Autodesk Inventor part; units mm, degrees
ref_plane "Work Plane3" through (-28.9586, -30.6315, -38.1) normal (-0.9063, 0.4226, 0) x (0, 0, 1)
ref_plane "Work Plane4" through (30.6491, -34.2567, 0.3) normal (0.9063, 0.4226, 0) x (0, 0, -1)
ref_plane "YZ Plane" through (0, 0, 0) normal (1, 0, 0) x (0, 1, 0)
sketch "Sketch19" plane through (0, 0, 0) normal (0, 0, 1) x (1, 0, 0)
  line L0 (47.55, -58) -> (-47.55, -58)
  line L1 (-100, -14) -> (156, -14) construction
  arc A0 (47.55, -58) -> (73.6817, -14) centre (0, 0) ccw
  arc A1 (-73.6817, -14) -> (-47.55, -58) centre (0, 0) ccw
  arc A2 (-64.7514, -20.7668) -> (-73.3933, -15.4412) centre (-66.5432, -14) ccw
  arc A3 (73.3933, -15.4412) -> (64.7514, -20.7668) centre (66.5432, -14) ccw
  arc A4 (-67.6299, -7.0849) -> (-64.8992, -20.3) centre (0, 0) ccw construction
  arc A5 (-64.7514, -20.7668) -> (-46.0869, -50) centre (0, 0) ccw
  arc A6 (46.0869, -50) -> (64.7514, -20.7668) centre (0, 0) ccw
  arc A7 (64.8058, -20.5962) -> (67.6299, -7.0849) centre (0, 0) ccw construction
  line L2 (0, 0) -> (-33.9351, 15.8242) construction
  line L3 (0, 0) -> (37.291, 17.3891) construction
  line L4 (0, 0) -> (0, -41) construction
  line L5 (0, 0) -> (-21.2237, -45.5143) construction
  line L6 (0, 0) -> (17.7082, -37.9755) construction
  line L7 (-12, -38.5394) -> (-12, -50)
  line L8 (12, -38.5394) -> (12, -50)
  line L9 (-26, -32.0111) -> (-26, -50)
  line L10 (26, -32.0111) -> (26, -50)
  line L11 (-18.4455, -35.5339) -> (-20.1359, -39.1591)
  line L12 (-20.1359, -39.1591) -> (-17.0545, -40.596)
  line L13 (-17.0545, -40.596) -> (-15.364, -36.9708)
  line L14 (15.364, -36.9708) -> (17.0545, -40.596)
  line L15 (17.0545, -40.596) -> (20.1359, -39.1591)
  line L16 (20.1359, -39.1591) -> (18.4455, -35.5339)
  line L17 (-12, -38.5394) -> (-15.364, -36.9708)
  line L18 (-18.4455, -35.5339) -> (-26, -32.0111)
  line L19 (12, -38.5394) -> (15.364, -36.9708)
  line L20 (18.4455, -35.5339) -> (26, -32.0111)
  line L21 (-46.0869, -50) -> (-26, -50)
  line L22 (-12, -50) -> (12, -50)
  line L23 (26, -50) -> (46.0869, -50)
  dimension "d378" = 58
  dimension "d379" = 14
  dimension "d381" = 75
  dimension "d383" = 75
  dimension "d384" = 14
  dimension "d385" = 14
  dimension "d389" = 25
  dimension "d390" = 25
  dimension "d391" = 90
  dimension "d392" = 90
  dimension "d393" = 24
  dimension "d394" = 12
  dimension "d395" = 14
  dimension "d396" = 14
  dimension "d399" = 3.4
  dimension "d400" = 4
  dimension "d401" = 1.7
  dimension "d402" = 3.4
  dimension "d403" = 1.7
  dimension "d404" = 4
extrude "Extrusion17" add sketch "Sketch19" along normal blind 140
sketch "Sketch20" plane through (0, 0, 0) normal (0, 0, -1) x (-1, 0, 0)
  line L0 (74, -50) -> (74, -58)
  line L1 (74, -58) -> (-74, -58)
  line L2 (-74, -58) -> (-74, -50)
  line L3 (47.55, -58) -> (-47.55, -58)
  line L4 (26, -50) -> (46.0869, -50)
  line L5 (-46.0869, -50) -> (-26, -50)
  line L6 (-26, -50) -> (-26, -32.0111)
  line L7 (-26, -32.0111) -> (-18.4455, -35.5339)
  line L8 (-18.4455, -35.5339) -> (-20.1359, -39.1591)
  line L9 (-20.1359, -39.1591) -> (-17.0545, -40.596)
  line L10 (-17.0545, -40.596) -> (-15.364, -36.9708)
  line L11 (-15.364, -36.9708) -> (-12, -38.5394)
  line L12 (-12, -38.5394) -> (-12, -50)
  line L13 (-12, -50) -> (12, -50)
  line L14 (12, -50) -> (12, -38.5394)
  line L15 (12, -38.5394) -> (15.364, -36.9708)
  line L16 (17.0545, -40.596) -> (20.1359, -39.1591)
  line L17 (20.1359, -39.1591) -> (18.4455, -35.5339)
  line L18 (18.4455, -35.5339) -> (26, -32.0111)
  line L19 (26, -32.0111) -> (26, -50)
  line L20 (26, -32.0111) -> (26, -50)
  line L21 (20.1359, -39.1591) -> (18.4455, -35.5339)
  line L22 (12, -50) -> (12, -38.5394)
  line L23 (12, -38.5394) -> (15.364, -36.9708)
  line L24 (15.364, -36.9708) -> (17.0545, -40.596)
  line L25 (15.364, -36.9708) -> (17.0545, -40.596)
  line L26 (-26, -50) -> (-26, -32.0111)
  line L27 (-12, -38.5394) -> (-12, -50)
  line L28 (-20.1359, -39.1591) -> (-17.0545, -40.596)
  line L29 (-17.0545, -40.596) -> (-15.364, -36.9708)
  line L30 (-15.364, -36.9708) -> (-12, -38.5394)
  line L31 (-26, -32.0111) -> (-18.4455, -35.5339)
  line L32 (-18.4455, -35.5339) -> (-20.1359, -39.1591)
  line L33 (-74, -50) -> (-26, -50)
  line L34 (-12, -50) -> (12, -50)
  line L35 (26, -50) -> (74, -50)
  point P0 (0, 0)
  dimension "d407" = 148
  dimension "d408" = 74
extrude "Extrusion18" add sketch "Sketch20" along normal blind 38.1
sketch "Sketch21" plane through (-12, -50, 140) normal (0, 1, 0) x (1, 0, 0)
  line L0 (48, 0) -> (-24, 0)
  line L1 (-24, 0) -> (-24, 12.7)
  line L2 (-24, 12.7) -> (48, 12.7)
  line L3 (48, 12.7) -> (48, 0)
  line L4 (48, 50.8) -> (-24, 50.8)
  line L5 (-24, 50.8) -> (-24, 76.2)
  line L6 (-24, 76.2) -> (48, 76.2)
  line L7 (48, 76.2) -> (48, 50.8)
  line L8 (48, 114.3) -> (-24, 114.3)
  line L9 (-24, 114.3) -> (-24, 139.7)
  line L10 (-24, 139.7) -> (48, 139.7)
  line L11 (48, 139.7) -> (48, 114.3)
  line L12 (24, 0) -> (0, 0)
  line L13 (38, 178.1) -> (38, 0)
  line L14 (-14, 178.1) -> (-14, 0)
  point P0 (12, 140)
  dimension "d412" = 10
  dimension "d413" = 10
  dimension "d414" = 12.7
  dimension "d415" = 38.1
  dimension "d416" = 25.4
  dimension "d417" = 38.1
  dimension "d418" = 25.4
extrude "Extrusion19" cut sketch "Sketch21" along normal up to next contours L0 L13 L2 L3 | L0 L14 L2 L13 | L14 L0 L1 L2 | L13 L6 L7 L4 | L4 L14 L6 L13 | L4 L5 L6 L14 | L13 L10 L11 L8 | L8 L14 L10 L13 | L8 L9 L10 L14
sketch "Sketch22" plane through (0, 0, 140) normal (0, 0, 1) x (1, 0, 0)
  arc A0 (-64.7514, -20.7668) -> (-73.3933, -15.4412) centre (-66.5432, -14) ccw
  circle A1 centre (-66.5432, -14) radius 3
  arc A2 (73.3933, -15.4412) -> (64.7514, -20.7668) centre (66.5432, -14) ccw
  circle A3 centre (66.5432, -14) radius 3
  arc A4 (-64.7514, -20.7668) -> (-46.0869, -50) centre (0, 0) ccw
  circle A5 centre (-46.0869, -50) radius 3
  arc A6 (46.0869, -50) -> (64.7514, -20.7668) centre (0, 0) ccw
  circle A7 centre (46.0869, -50) radius 3
  dimension "d421" = 6
  dimension "d422" = 6
  dimension "d423" = 6
  dimension "d424" = 6
extrude "Extrusion20" add sketch "Sketch22" along normal blind 20 and the other way blind 10
fillet "Fillet1" radius 0.5 4 edges at (-69.5432, -14, 160) (-49.0869, -50, 160) (43.0869, -50, 160) (63.5432, -14, 160)
sketch "Sketch23" plane through (55.9017, -50, 0) normal (0, 1, 0) x (1, 0, 0)
  circle A0 centre (-115.9017, 26.1) radius 1.3
  line L0 (-129.9017, 0) -> (-129.9017, 38.1)
  line L1 (18.0983, 0) -> (18.0983, 38.1)
  line L2 (-129.9017, 38.1) -> (-81.9017, 38.1)
  line L3 (-29.9017, 38.1) -> (18.0983, 38.1)
  circle A1 centre (-55.9017, 26.1) radius 3.25
  line L4 (-67.9017, 38.1) -> (-43.9017, 38.1)
  circle A2 centre (8.0983, 26.1) radius 3.25
  point P0 (-55.9017, 0)
  dimension "d430" = 2.6
  dimension "d431" = 14
  dimension "d433" = 12
  dimension "d435" = 6.5
  dimension "d436" = 0
  dimension "d437" = 12
  dimension "d453" = 6.5
  dimension "d454" = 12
  dimension "d455" = 10
extrude "Extrusion21" cut sketch "Sketch23" against normal through all
ref_plane "Work Plane3" through (-28.9586, -30.6315, -38.1) normal (-0.9063, 0.4226, 0) x (0, 0, 1)
sketch "Sketch24" plane through (-28.9586, -30.6315, -38.1) normal (-0.9063, 0.4226, 0) x (0, 0, 1)
  circle A0 centre (19.05, -2.5) radius 0.75
  line L0 (0, 0) -> (38.4, 0)
  line L1 (0, -16.3035) -> (0, 0)
  point P0 (38.1, 40)
  dimension "d441" = 1.5
  dimension "d442" = 2.5
  dimension "d443" = 19.05
extrude "Extrusion22" cut sketch "Sketch24" against normal blind 12
ref_plane "Work Plane4" through (30.6491, -34.2567, 0.3) normal (0.9063, 0.4226, 0) x (0, 0, -1)
sketch "Sketch25" plane through (30.6491, -34.2567, 0.3) normal (0.9063, 0.4226, 0) x (0, 0, -1)
  circle A0 centre (19.35, 1.5) radius 0.75
  line L0 (38.4, 4) -> (38.4, -12.3035)
  line L1 (38.4, 4) -> (0, 4)
  point P0 (0.3, 44)
  dimension "d447" = 19.05
  dimension "d448" = 1.5
  dimension "d450" = 2.5
extrude "Extrusion23" cut sketch "Sketch25" against normal blind 12
sketch "Sketch26" plane through (55.9017, -50, 0) normal (0, 1, 0) x (1, 0, 0)
  line L0 (-45.9017, -92) -> (-45.9017, -48)
  line L1 (-65.9017, -48) -> (-65.9017, -92)
  arc A0 (-65.9017, -92) -> (-45.9017, -92) centre (-55.9017, -92) ccw
  arc A1 (-45.9017, -48) -> (-65.9017, -48) centre (-55.9017, -48) ccw
  line L2 (-12.8148, -140) -> (-98.9886, -140)
  point P0 (-55.9017, 0)
  dimension "d456" = 20
  dimension "d457" = 10
  dimension "d458" = 44
extrude "Extrusion24" cut sketch "Sketch26" against normal through all
sketch "Sketch27" plane through (0, 0, -38.1) normal (0, 0, -1) x (-1, 0, 0)
  line L0 (-74, -50) -> (-74, -58)
  line L1 (-74, -58) -> (74, -58)
  line L2 (74, -58) -> (74, -50)
  line L3 (74, -50) -> (26, -50)
  line L4 (26, -50) -> (26, -32.0111)
  line L5 (26, -32.0111) -> (18.4455, -35.5339)
  line L6 (18.4455, -35.5339) -> (20.1359, -39.1591)
  line L7 (20.1359, -39.1591) -> (17.0545, -40.596)
  line L8 (17.0545, -40.596) -> (15.364, -36.9708)
  line L9 (15.364, -36.9708) -> (12, -38.5394)
  line L10 (12, -38.5394) -> (12, -50)
  line L11 (12, -50) -> (-12, -50)
  line L12 (-12, -50) -> (-12, -38.5394)
  line L13 (-12, -38.5394) -> (-15.364, -36.9708)
  line L14 (-15.364, -36.9708) -> (-17.0545, -40.596)
  line L15 (-17.0545, -40.596) -> (-20.1359, -39.1591)
  line L16 (-20.1359, -39.1591) -> (-18.4455, -35.5339)
  line L17 (-18.4455, -35.5339) -> (-26, -32.0111)
  line L18 (-26, -32.0111) -> (-26, -50)
  line L19 (-26, -50) -> (-74, -50)
  line L20 (-74, -50) -> (-74, -58)
  line L21 (74, -50) -> (55.9017, -50)
  line L22 (-74, -58) -> (74, -58)
  line L23 (74, -58) -> (74, -50)
  line L24 (74, -50) -> (-74, -50)
  line L25 (-74, -50) -> (-74, -58)
  point P0 (0, 0)
extrude "Extrusion25" add sketch "Sketch27" along normal blind 9.15 contours L19 L24 L11 L3 L2 L1 L0
sketch "Sketch28" plane through (-74, -50, 0) normal (0, 1, 0) x (1, 0, 0)
  line L0 (109, 42.25) -> (39, 42.25) construction
  line L1 (39, 42.25) -> (39, 11.25) construction
  line L2 (39, 11.25) -> (109, 11.25) construction
  line L3 (109, 11.25) -> (109, 42.25) construction
  line L4 (0, 47.25) -> (148, 47.25) construction
  point P0 (74, 0)
  point P1 (74, 42.25)
  point P2 (74, 47.25)
  dimension "d464" = 70
  dimension "d465" = 31
  dimension "d466" = 5
hole "Hole1" at (35, -50, -11.25) at (35, -50, -42.25) at (-35, -50, -42.25) at (-35, -50, -11.25) direction (0, -1, 0) diameter 4.5 end through all
equation "\"BendRadius\" = Thickness"
equation "\"BendReliefWidth\" = Thickness"
equation "\"BendReliefDepth\" = 0.5 * Thickness"
equation "\"CornerReliefSize\" = 4 * Thickness"
equation "\"MinimumRemnant\" = 2 * Thickness"
equation "\"TransitionRadius\" = BendRadius"
equation "\"JacobiRadiusSize\" = BendRadius"
equation "\"GapSize\" = Thickness"
properties part number "3214_Bed Rail End_V1" material "Acetal Resin, White"
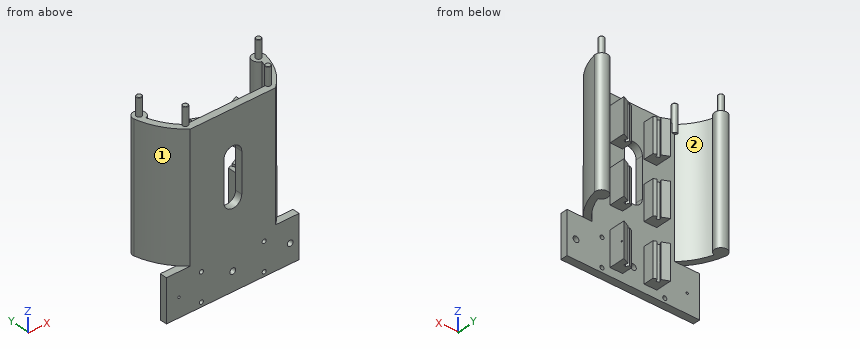
Model file for the job. Use its own axes, mm. Face numbers are marked on the shaded views. Give positions to 0.01 mm unless a question says otherwise; leave off trailing zeros. Order: outer loops, then holes, each group sorted by start corner. A loop starts at its lowest first (then second) coordinate and runs counter-clockwise, first axis right, second up. Notation, with made-up numbers: (59, 23.25) - (109, 23.25) arc R28 ccw to (109, 51.25) - close; hole circle Ø5 at (-16.5, -11). An arc over 180 degrees is marked (long way). Return JSON: item names as keys, results as strings.
1) Flat gauge pins, fed straight in: P1, Ø8, axis at x = -38, z = 49, coming from the +Y side; P2, Ø5.5, axis at y = -39.5, z = 53, coming from the +X side; P3, Ø10, axis at x = -13.5, z = 37.5, coming from the +Y side; P4, Ø12, axis at x = 49.5, y = -19, coming from the -Z side. Where does each tip first touch, or does it go through?
Geometry says:
{"P1": "y = -50", "P2": "x = 65.38", "P3": "y = -35.51", "P4": "through"}
2) Cut at B-B, the plane x = -35. Give the cut face in (y, z).
Geometry says:
{"outline": "(-58, -47.25) - (-50, -47.25) - (-50, -44.5) - (-58, -44.5) - close; (-58, -40) - (-50, -40) - (-50, -13.5) - (-58, -13.5) - close; (-58, -9) - (-50, -9) - (-50, 140) - (-58, 140) - close"}
3) Cut at A-A, the plane z = -42.25. Give the cut face in (x, y).
Geometry says:
{"outline": "(-74, -58) - (-37.25, -58) - (-37.25, -50) - (-74, -50) - close; (-32.75, -58) - (32.75, -58) - (32.75, -50) - (-32.75, -50) - close; (37.25, -58) - (74, -58) - (74, -50) - (37.25, -50) - close"}
4) Probe line 1 (Z direction, x = 35, y = -52.25); line 2 (X direction, y = -55, z = -11); line 3 (X direction, y = -52.5, z = -26.1). List the from-to ranges inside material, lowest first. Write a range as from..to.
Geometry says:
{"line 1": "-47.25..-44.5, -40..-13.5, -9..140", "line 2": "-74..-37.24, -32.76..32.76, 37.24..74", "line 3": "-74..-61.3, -58.7..-3.25, 3.25..60.75, 67.25..74"}
5) Pull direction Y, two halves, no side cores. Call the marked faces 1 and 2: pulls with the +Y half, pulls with the -Y half, needs draft (parallel to the pull), parting line crosses it, or undercut.
Geometry says:
{"face 1": "pulls with the -Y half", "face 2": "undercut"}
6) Cut at C-C, the plane y = -27.5. Give the cut face in (x, z), plus the area to 3 significant figures.
Geometry says:
{"outline": "(-69.78, 0) - (-62.19, 0) - (-62.19, 140) - (-69.78, 140) - close; (62.19, 0) - (69.78, 0) - (69.78, 140) - (62.19, 140) - close", "area": "2,120 mm²"}
